from build123d import *

# Parameters (mm, degrees)
SALIENTE_EXTRUIR1_DEPTH = 1.5
CROQUIS2_W              = 30
CROQUIS2_H              = 3.1
CORTAR_EXTRUIR1_DEPTH   = 10
CROQUIS6_R              = 1.25
CROQUIS6_R_2            = 4.5
CORTAR_EXTRUIR2_DEPTH   = 3


with BuildPart() as part:
    # Croquis1 → Saliente-Extruir1 (new, symmetric)
    with BuildSketch(Plane.XY):
        Polygon((-100, -27), (-100, -45), (-71.428571429, -45), (-71.428571429, -41.9), (-42.857142857, -41.9), (-42.857142857, -45), (-14.285714286, -45), (-14.285714286, -41.9), (14.285714286, -41.9), (14.285714286, -45), (42.857142857, -45), (42.857142857, -41.9), (71.428571429, -41.9), (71.428571429, -45), (100, -45), (100, -27), (96.9, -27), (96.9, -9), (100, -9), (100, 9), (96.9, 9), (96.9, 27), (100, 27), (100, 45), (71.428571429, 45), (71.428571429, 41.9), (42.857142857, 41.9), (42.857142857, 45), (14.285714286, 45), (14.285714286, 41.9), (-14.285714286, 41.9), (-14.285714286, 45), (-42.857142857, 45), (-42.857142857, 41.9), (-71.428571429, 41.9), (-71.428571429, 45), (-100, 45), (-100, 27), (-96.9, 27), (-96.9, 9), (-100, 9), (-100, -9), (-96.9, -9), (-96.9, -27), align=None)
    extrude(amount=SALIENTE_EXTRUIR1_DEPTH, both=True)

    # Croquis2 → Cortar-Extruir1 (cut)
    with BuildSketch(Plane.XY.offset(1.5)):
        with Locations((-60, -25.45)):
            Rectangle(CROQUIS2_W, CROQUIS2_H)
        with Locations((60, -25.45)):
            Rectangle(CROQUIS2_W, CROQUIS2_H)
    extrude(amount=-CORTAR_EXTRUIR1_DEPTH, mode=Mode.SUBTRACT)

    # Croquis6 → Cortar-Extruir2 (cut)
    with BuildSketch(Plane(origin=(0, 0, -1.5), x_dir=(-1, 0, 0), z_dir=(0, 0, -1))):
        with Locations((53.253279384, 30)):
            Circle(CROQUIS6_R)
        with Locations((73.053279384, 30)):
            Circle(CROQUIS6_R)
        with Locations((58.753279384, 33)):
            Circle(CROQUIS6_R_2)
    extrude(amount=-CORTAR_EXTRUIR2_DEPTH, mode=Mode.SUBTRACT)


solid = part.part
Work out the finished part from the listing and answer in its coordinate system (mm). Give positions to 0.01 mm unless a question says otherwise; leave off trailing zeros. Write each loop counter-clockwise with the first axis right and the second up, starting at its lowest first coordinate (ties: lowest second). Pieces come first, ordered by that corner, then holes. Notation, with made-up numbers: (3, 30.5) - (15, 30.5) arc R12 ccw to (15, 49.5) - close; hole circle Ø5 at (66.5, 79.5). An arc over 180 degrees is marked (long way). One line per item, written item: value. Start each with the question number.
1. Find section B-B (x = -57.5). Write down the section's boundary in (y, z).
2. Consider probe 1 along Y at (x, z) = (-53, -0.05); probe 2 along Y at (x, z) = (-62, -1.2); probe 3 along Y at (x, z) = (47, 0.4). Determine where each line is inside the solid, lowest interval first.
3. Find section D-D (y = 14). Write down the section's boundary in (x, z).
4. Find section C-C (z = 0.8). State how many separate pieces and enclosed holes the cut face has, then the cut area to 3 significant figures.
5. Find section A-A (x = 61). Write down the section's boundary in (y, z), then the cut area to 3 significant figures.
6. For a pull along Y with two mould halves and no side action, classify faces 1 (the flat face through (-1, 1, -1.5)), 2 (the cylindrical face through (-60.83, 29.01, -0.02)) as +Y half, -Y half, draft (parallel to the pull), parting line (faces both ways), or undercut.
7. Given pin 1 (0.9 mm diameter, centred on y = -25.5, z = -0.5, fed in from +X); pin 2 (0.9 mm diameter, centred on y = -15.5, z = 0, fed in from -X); pin 3 (1 mm diameter, centred on x = -7, z = -0.5, fed in from +Y), each flat-ended and moving along its own axis, determine where each tip first touches the part or whether it passes through.
Geometry results:
1. outline: (-41.9, -1.5) - (-27, -1.5) - (-27, 1.5) - (-41.9, 1.5) - close; (-23.9, -1.5) - (28.68, -1.5) - (28.68, 1.5) - (-23.9, 1.5) - close; (37.32, -1.5) - (41.9, -1.5) - (41.9, 1.5) - (37.32, 1.5) - close
2. probe 1: -41.9 to -27, -23.9 to 28.78, 31.22 to 41.9
2. probe 2: -41.9 to -27, -23.9 to 29.88, 36.12 to 41.9
2. probe 3: -41.9 to -27, -23.9 to 41.9
3. outline: (-96.9, -1.5) - (96.9, -1.5) - (96.9, 1.5) - (-96.9, 1.5) - close
4. separate pieces: 1
4. enclosed holes: 5
4. area: 17,000 mm2
5. outline: (-41.9, -1.5) - (-27, -1.5) - (-27, 1.5) - (-41.9, 1.5) - close; (-23.9, -1.5) - (41.9, -1.5) - (41.9, 1.5) - (-23.9, 1.5) - close
5. area: 242 mm2
6. face 1: draft
6. face 2: undercut
7. pin 1: x = 96.9
7. pin 2: x = -96.9
7. pin 3: y = 41.9
